The model under review builds one solid part; all positions refer to its coordinate system, in mm. A direction names the side the tool comes from. Give positions to 0.01 mm unless a question says otherwise; leave off trailing zeros. Write each loop counter-clockwise with the first axis right and the second up, starting at its lowest first coordinate (ties: lowest second). Pieces come first, ordered by that corner, then holes. Notation, with made-up numbers: (60, 54.25) - (91, 54.25) arc R12 cw to (91, 73.25) - close; hole circle Ø10 at (-14.75, 80). An arc over 180 degrees is marked (long way). Write item = value, one per line.
```python
from build123d import *

# Parameters (mm, degrees)
SKETCH1_R           = 6.04
SKETCH1_R_2         = 2.54
SKETCH1_R_3         = 9.525
SKETCH1_R_4         = 2.07
BOSS_EXTRUDE1_DEPTH = 0.875
FILLET2_R           = 10


with BuildPart() as part:
    # Sketch1 → Boss-Extrude1 (new, symmetric)
    # profile 1 of 5: a face of its own
    with BuildSketch(Plane.XY):
        with Locations((16.38, 50.8)):
            Circle(SKETCH1_R)
        with Locations((16.38, 50.8)):
            Circle(SKETCH1_R_2, mode=Mode.SUBTRACT)
    # profile 2 of 5: a face of its own
    with BuildSketch(Plane.XY):
        with Locations((0, 25.4)):
            Circle(SKETCH1_R_3)
        with Locations((0, 25.4)):
            Circle(SKETCH1_R_4, mode=Mode.SUBTRACT)
    # profile 3 of 5: a face of its own
    with BuildSketch(Plane.XY):
        with BuildLine():
            ThreePointArc((-7.356213705, 31.450763995), (3.213852008, 34.366425167), (9.525, 25.4))
            Line((9.525, 25.4), (21.694295801, 47.929484342))
            ThreePointArc((21.694295801, 47.929484342), (13.010594873, 45.787145615), (11.715272359, 54.636914912))
            Line((11.715272359, 54.636914912), (-7.356213705, 31.450763995))
        make_face()
    # profile 4 of 5: a face of its own
    with BuildSketch(Plane.XY):
        with BuildLine():
            Line((9.525, 0), (9.525, 25.4))
            ThreePointArc((9.525, 25.4), (0, 15.875), (-9.525, 25.4))
            Line((-9.525, 25.4), (-9.525, 0))
            ThreePointArc((-9.525, 0), (0, 9.525), (9.525, 0))
        make_face()
        with Locations((0, 12.7)):
            Circle(SKETCH1_R_4, mode=Mode.SUBTRACT)
    # profile 5 of 5: a face of its own
    with BuildSketch(Plane.XY):
        Circle(SKETCH1_R_3)
        Circle(SKETCH1_R_4, mode=Mode.SUBTRACT)
    extrude(amount=BOSS_EXTRUDE1_DEPTH, both=True)

    # Fillet2
    fillet2_edges = [part.edges().sort_by_distance(p)[0] for p in [
        (9.525, 25.4, 0),
    ]]
    fillet(fillet2_edges, radius=FILLET2_R)


solid = part.part
```
1. Take a section at B-B on x = -1. Give the boundary of the cut face in (y, z) (3 decimals), and give its area (3 significant figures).
Findings below:
outline = (-9.472, -0.875) - (-1.812, -0.875) - (-1.812, 0.875) - (-9.472, 0.875) - close; (1.812, -0.875) - (10.888, -0.875) - (10.888, 0.875) - (1.812, 0.875) - close; (14.512, -0.875) - (23.588, -0.875) - (23.588, 0.875) - (14.512, 0.875) - close; (27.212, -0.875) - (39.178, -0.875) - (39.178, 0.875) - (27.212, 0.875) - close
area = 66.1 mm²
2. For line 1 (Y direction, x = 0, z = -0.2) (3 decimals); line 2 (Y direction, x = 15, z = -0.6); line 3 (X direction, y = 4, z = 0.75) (3 decimals), list the stretches that pass through material, from the lowest coordinate up. Write a range as from..to.
Findings below:
line_1 = -9.525..-2.07, 2.07..10.63, 14.77..23.33, 27.47..40.394
line_2 = 35.54..48.67, 52.93..56.68
line_3 = -9.525..9.525
3. Take a section at D-D on x = 6. Give the boundary of the cut face in (y, z) (3 decimals), and give its area (3 significant figures).
Findings below:
outline = (-7.398, -0.875) - (47.689, -0.875) - (47.689, 0.875) - (-7.398, 0.875) - close
area = 96.4 mm²
4. Insertion check: P1, Ø0.9, axis at y = 15.5, z = -0.5, coming from the +X side (3 decimals); P2, Ø1, axis at y = 45, z = 0.5, coming from the -X side. Each pin has a flat end and moves straight along its axis. Give the tip position at first contact, or say it passes through.
Findings below:
P1 = 9.525
P2 = 3.38
5. Take a section at A-A on x = 16.38. Give the boundary of the cut face in (y, z) (3 decimals), and give its area (3 significant figures).
Findings below:
outline = (38.091, -0.875) - (48.26, -0.875) - (48.26, 0.875) - (38.091, 0.875) - close; (53.34, -0.875) - (56.84, -0.875) - (56.84, 0.875) - (53.34, 0.875) - close
area = 23.9 mm²
6. Take a section at C-C on y = 22. Give the boundary of the cut face in (x, z) (3 decimals), and give its area (3 significant figures).
Findings below:
outline = (-9.525, -0.875) - (9.525, -0.875) - (9.525, 0.875) - (-9.525, 0.875) - close
area = 33.3 mm²
7. Machinability: for faces 1 (the flat face through (9.525, 11, 0)), 2 (the flat face through (3, 24, -0.875)), which of the approach directions +Z, -Z, +X, -X, +Y, -Y give a long, thin tool a straight path to every point of the face, cutting with its end or side? Answer none if there is none.
Findings below:
face_1 = +Z, -Z, +X, -Y
face_2 = -Z, +X, -X, +Y, -Y
